```python
from build123d import *

# Parameters (mm, degrees)
F1_R     = 4.7625
F2_DEPTH = 50.8
F0_R     = 38.1
F0_R_2   = 28.8036
F3_DEPTH = 304.8
F4_DEPTH = 304.8


with BuildPart() as f2:
    # F1 (on Right) → F2 (new body)
    with BuildSketch(Plane.YZ):
        with Locations((-19.05, 0)):
            Circle(F1_R)
    extrude(amount=F2_DEPTH)

    # F0 (on Front) → F3 (join)
    with BuildSketch(Plane.XZ):
        Circle(F0_R)
        Circle(F0_R_2, mode=Mode.SUBTRACT)
        Circle(F0_R_2)
    extrude(amount=F3_DEPTH)

    # F0 (on Front) → F4 (cut)
    with BuildSketch(Plane.XZ):
        Circle(F0_R_2)
    extrude(amount=F4_DEPTH, mode=Mode.SUBTRACT)

    # F5: F2 across face


with BuildPart() as f2_1:
    add(f2.part)
    add(f2.part.mirror(Plane.XZ.offset(304.8)))


solid = f2_1.part
```
CAD build for the part. Positions are in the model's coordinates, mm. A direction names the side the tool comes from. Round coordinates to 2 decimals unless told otherwise and drop trailing zeros. Order: outer loops, then holes, each group sorted by start corner. A loop starts at its lowest first (then second) coordinate and runs counter-clockwise, first axis right, second up.
Item 1: Saw through at A-A on x = 0. Write the cut outline in (y, z), then the cut area to 3 significant figures.
Item 2: Probe line 1 along Z through (x, y) = (0, -463); line 2 along Z through (x, y) = (-2, -337); line 3 along X through (y, z) = (-203.5, 8). List the from-to ranges inside material, lowest first.
Item 3: Saw through at C-C on y = -169. Write the cut outline in (x, z).
Item 4: Tool access for faces 1 (the face through (44.2, -14.5, 1.4)), 2 (the face through (50.8, -19, 0)): list every direction of +Z, -Z, +X, -X, +Y, -Y with a clear straight run to the whole face (end or side of a thin tool).
Item 5: Mould opens along Z. For faces 3 (the face through (13.291, -309.067, -25.554)), 4 (the face through (-30.235, -309.067, -23.183)), 5 (the face through (-14, -609.6, 26)) say: pulls with the +Z half, pulls with the -Z half, needs draft (parallel to the pull), parting line crosses it, or undercut.
Item 6: Saw through at B-B on z = 21.5. Write the cut outline in (x, y), then the cut area to 3 significant figures.
Item 7: Pin check, flat tips, straight feed: pin 1 (5 mm diameter, centred on x = 17.5, y = -480, fed in from +Z); pin 2 (1.5 mm diameter, centred on x = -21, z = 18, fed in from +Y); pin 3 (2 mm diameter, centred on y = -452.5, z = -10, fed in from -X); pin 4 (12 mm diameter, centred on x = 32, y = -91, fed in from -Z). Stop position of each tip, or through.
Reported:
1. outline: (-609.6, -38.1) - (0, -38.1) - (0, -28.8) - (-609.6, -28.8) - close; (-609.6, 28.8) - (0, 28.8) - (0, 38.1) - (-609.6, 38.1) - close
1. area: 11,300 mm2
2. line 1: z = -38.1 to -28.8, 28.8 to 38.1
2. line 2: z = -38.05 to -28.73, 28.73 to 38.05
2. line 3: x = -37.25 to -27.67, 27.67 to 37.25
3. outline: circle Ø76.2 at (0, 0); hole circle Ø57.61 at (0, 0)
4. face 1: +X
4. face 2: +Z, -Z, +X, +Y, -Y
5. face 3: undercut
5. face 4: parting line crosses it
5. face 5: needs draft
6. outline: (-31.45, -609.6) - (-19.17, -609.6) - (-19.17, 0) - (-31.45, 0) - close; (19.17, -609.6) - (31.45, -609.6) - (31.45, 0) - (19.17, 0) - close
6. area: 15,000 mm2
7. pin 1: stops at z = 35.02
7. pin 2: passes through
7. pin 3: stops at x = -37.02
7. pin 4: stops at z = -27.85
